CAD build for the part. Positions are in the model's coordinates, mm. A direction names the side the tool comes from. Give positions to 0.01 mm unless a question says otherwise; leave off trailing zeros. Order: outer loops, then holes, each group sorted by start corner. A loop starts at its lowest first (then second) coordinate and runs counter-clockwise, first axis right, second up.
Item 1: Which spindle directions (+Z, -Z, +X, -X, +Y, -Y) get a long thin tool onto all of the face, cutting with end or side? Do faces 1 (the flat face through (15, 3, 82)), 2 (the flat face through (74, 5, -8.762)), 3 (the flat face through (105, 5, 1.238)). Say none if no direction does.
Item 2: Band-saw the part on B-B on z = 119. Count the separate pieces of the cut face and the enclosed holes in it, plus the area to 3 significant figures.
Item 3: Band-saw the part on A-A on x = 103. Give the cut face in (y, z).
Item 4: Wall check: L1, parallel to X at y = 2.5, z = 67; L2, parallel to Z at x = 62, y = 1.75; L3, parallel to Z at x = 138.5, y = 6. Give the ranges that are in metal, low to high.
Item 5: Two-plate mould, pull along Z, no slides. Class faces 4 (the flat face through (74, 5, 171.238)), 5 (the flat face through (143.304, 2.7, 82.5)), 6 (the flat face through (8, 7, 82)): released by +Z, released by -Z, zero draft, split by the parting line, or undercut.
```python
from build123d import *

# Parameters (mm, degrees)
SKETCH1_W           = 137.099988832
SKETCH1_H           = 180
BOSS_EXTRUDE1_DEPTH = 10
SKETCH2_W           = 150
SKETCH2_H           = 4
CUT_EXTRUDE1_DEPTH  = 160


with BuildPart() as part:
    # Sketch1 → Boss-Extrude1 (new body)
    with BuildSketch(Plane(origin=(0, 0, 0), x_dir=(1, 0, 0), z_dir=(0, 1, 0))):
        with Locations((74.75359819, -81.23781213)):
            Rectangle(SKETCH1_W, SKETCH1_H)
        with BuildLine():
            Line((16.203603774, -1.23781213), (72.1788033, -1.23781213))
            ThreePointArc((72.1788033, -1.23781213), (72.355579995, -1.164588825), (72.4288033, -0.98781213))
            Line((72.4288033, -0.98781213), (72.4288033, 3.51218787))
            ThreePointArc((72.4288033, 3.51218787), (72.502026605, 3.688964566), (72.6788033, 3.76218787))
            Line((72.6788033, 3.76218787), (77.1788033, 3.76218787))
            ThreePointArc((77.1788033, 3.76218787), (77.355579995, 3.688964566), (77.4288033, 3.51218787))
            Line((77.4288033, 3.51218787), (77.4288033, -0.98781213))
            ThreePointArc((77.4288033, -0.98781213), (77.502026605, -1.164588825), (77.6788033, -1.23781213))
            Line((77.6788033, -1.23781213), (133.303592606, -1.23781213))
            Line((133.303592606, -1.23781213), (133.303592606, -161.23781213))
            Line((133.303592606, -161.23781213), (77.6788033, -161.23781213))
            ThreePointArc((77.6788033, -161.23781213), (77.502026605, -161.311035434), (77.4288033, -161.48781213))
            Line((77.4288033, -161.48781213), (77.4288033, -165.98781213))
            ThreePointArc((77.4288033, -165.98781213), (77.355579995, -166.164588825), (77.1788033, -166.23781213))
            Line((77.1788033, -166.23781213), (72.6788033, -166.23781213))
            ThreePointArc((72.6788033, -166.23781213), (72.502026605, -166.164588825), (72.4288033, -165.98781213))
            Line((72.4288033, -165.98781213), (72.4288033, -161.48781213))
            ThreePointArc((72.4288033, -161.48781213), (72.355579995, -161.311035434), (72.1788033, -161.23781213))
            Line((72.1788033, -161.23781213), (16.203603774, -161.23781213))
            Line((16.203603774, -161.23781213), (16.203603774, -1.23781213))
        make_face(mode=Mode.SUBTRACT)
        with BuildLine():
            Line((9.203603774, -154.23781213), (9.203603774, -8.23781213))
            ThreePointArc((9.203603774, -8.23781213), (11.203603774, -6.23781213), (13.203603774, -8.23781213))
            Line((13.203603774, -8.23781213), (13.203603774, -154.23781213))
            ThreePointArc((13.203603774, -154.23781213), (11.203603774, -156.23781213), (9.203603774, -154.23781213))
        make_face(mode=Mode.SUBTRACT)
        with BuildLine():
            Line((136.303592606, -154.23781213), (136.303592606, -8.23781213))
            ThreePointArc((136.303592606, -8.23781213), (138.303592606, -6.23781213), (140.303592606, -8.23781213))
            Line((140.303592606, -8.23781213), (140.303592606, -154.23781213))
            ThreePointArc((140.303592606, -154.23781213), (138.303592606, -156.23781213), (136.303592606, -154.23781213))
        make_face(mode=Mode.SUBTRACT)
    extrude(amount=BOSS_EXTRUDE1_DEPTH)

    # Sketch2 → Cut-Extrude1 (cut)
    with BuildSketch(Plane(origin=(143.303592606, 0, 0), x_dir=(0, 0, -1), z_dir=(1, 0, 0))):
        with Locations((-81.23781213, 5)):
            Rectangle(SKETCH2_W, SKETCH2_H)
    extrude(amount=-CUT_EXTRUDE1_DEPTH, mode=Mode.SUBTRACT)


solid = part.part
```
The answers:
1. face 1: +X, -X
1. face 2: -Z, +X, -X, +Y, -Y
1. face 3: +Y, -Y
2. separate pieces: 8
2. enclosed holes: 0
2. area: 72.0 mm2
3. outline: (0, -8.76) - (10, -8.76) - (10, 1.24) - (0, 1.24) - close; (0, 161.24) - (10, 161.24) - (10, 171.24) - (0, 171.24) - close
4. L1: x = 6.2 to 9.2, 13.2 to 16.2, 133.3 to 136.3, 140.3 to 143.3
4. L2: z = -8.76 to 1.24, 161.24 to 171.24
4. L3: z = -8.76 to 6.24, 156.24 to 171.24
5. face 4: released by +Z
5. face 5: zero draft
5. face 6: undercut
